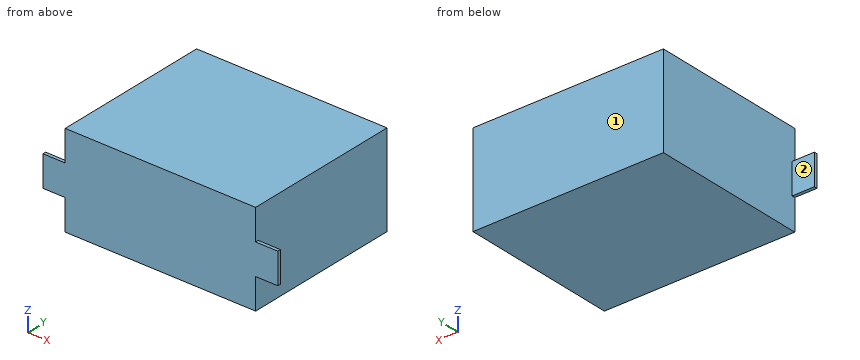
Autodesk Inventor part; units mm, degrees
ref_plane "YZ Plane" through (0, 0, 0) normal (1, 0, 0) x (0, 1, 0)
ref_plane "XZ Plane" through (0, 0, 0) normal (0, 1, 0) x (-1, 0, 0)
ref_plane "XY Plane" through (0, 0, 0) normal (0, 0, 1) x (1, 0, 0)
sketch "Skizze1" plane through (0, 0, 0) normal (0, 0, 1) x (1, 0, 0)
  line L0 (30, -25) -> (-30, -25)
  line L1 (-30, -25) -> (-30, 25)
  line L2 (-30, 25) -> (30, 25)
  line L3 (30, 25) -> (30, -25)
  point P0 (0, 0)
  point P1 (-30, 0)
  point P2 (0, 25)
  dimension "d0" = 50
  dimension "d1" = 60
extrude "Extrusion1" add sketch "Skizze1" against normal blind 29.1
sketch "Skizze4" plane through (30, -25, 0) normal (1, 0, 0) x (0, 0, -1)
  line L0 (0, 0) -> (0, 50)
  line L1 (0, 0) -> (29.1, 0)
  line L2 (29.1, 0) -> (19.4, 0)
  line L3 (9.7, 0) -> (19.4, 0)
  line L4 (19.4, 0) -> (19.4, 1)
  line L5 (19.4, 1) -> (9.7, 1)
  line L6 (9.7, 1) -> (9.7, 0)
  point P0 (0, 25)
extrude "Extrusion3" add sketch "Skizze4" along normal blind 7
mirror "Spiegeln1" about plane through (0, 0, 0) normal (1, 0, 0) of "Extrusion3"
sketch "Skizze5" plane through (30, -24, -9.7) normal (0, 1, 0) x (1, 0, 0)
  line L0 (7, 0) -> (7, 9.7)
  line L1 (0, -9.7) -> (0, 19.4)
  line L2 (0, -9.7) -> (0, 0)
  line L3 (-60, 9.7) -> (-60, 0)
  line L4 (-60, 9.7) -> (-67, 9.7)
  line L5 (-67, 9.7) -> (-67, 0)
  point P0 (-30, -9.7)
  point P1 (3.5, 4.7412)
  point P2 (-63.5, 4.85)
sketch "Skizze6" plane through (-30, 25, 0) normal (0, 1, 0) x (1, 0, 0)
  line L0 (22.3981, 26.7886) -> (69.5939, 26.7886) construction
  line L1 (69.5939, 26.7886) -> (69.5939, 22.4356) construction
  line L2 (69.5939, 22.4356) -> (22.3981, 22.4356) construction
  line L3 (22.3981, 22.4356) -> (22.3981, 26.7886) construction
  point P0 (30, 0)
properties part number "Akku1" material "Gold"
Could you check a few things on this model? Use its own coordinates, in mm. Face numbers are marked on the shaded views. A direction names the side the tool comes from. Coordinates: 2 decimals unless noted, no trailing zeros. Write each loop counter-clockwise with the first axis right and the second up, starting at its lowest first coordinate (ties: lowest second). Pieces come first, ordered by that corner, then holes. Notation, with made-up numbers: (5, 2.25) -> (27, 2.25) arc R18 ccw to (27, 17.25) -> close; hole circle Ø10 at (42.25, -1.5). An arc over 180 degrees is marked (long way). Return JSON: item names as keys, results as strings.
(1) Imagine slicing it at B-B, the plane z = -26.25. Please give me the cut outline in (x, y), then the cut area to 3 significant figures.
Numbers:
{"outline": "(-30, -25) -> (30, -25) -> (30, 25) -> (-30, 25) -> close", "area": "3,000 mm2"}
(2) I'm going to push flat-ended pins straight in: pin 1 (5.5 mm diameter, centred on x = -34.5, z = -13, fed in from +Y); pin 2 (8.5 mm diameter, centred on y = 11.5, z = -19, fed in from +X); pin 3 (1.1 mm diameter, centred on x = -34, y = -24.5, fed in from -Z). Where does each tip first touch, or does it pass through?
Numbers:
{"pin 1": "stops at y = -24", "pin 2": "stops at x = 30", "pin 3": "stops at z = -19.4"}
(3) I need wall thicknesses on L1, parallel to X at y = 9, z = -23.5; L2, parallel to Y at x = 33, z = -11.75. Which ranges of each line are inside material? Lowest first, please.
Numbers:
{"L1": "x = -30 to 30", "L2": "y = -25 to -24"}
(4) Imagine slicing it at A-A, the plane y = -20. Please give me the cut outline in (x, z), then the cut area to 3 significant figures.
Numbers:
{"outline": "(-30, -29.1) -> (30, -29.1) -> (30, 0) -> (-30, 0) -> close", "area": "1,750 mm2"}
(5) Which directions (+Z, -Z, +X, -X, +Y, -Y) give clear straight access to the entire face, cutting with the end or side of a thin tool? Please do the marked faces 1 and 2.
Numbers:
{"face 1": "+Z, -Z, +X, -X, +Y", "face 2": "+Z, -Z, -X, +Y"}
